Build history of the part. All positions in model axes, mm. Coordinates: 2 decimals unless noted, no trailing zeros. Loops run counter-clockwise (first coordinate to the right, second up) from the corner with the lowest first, then second, coordinate; pieces in that order, holes last.
Item 1: Flat gauge pins, fed straight in: pin 1 (1 mm diameter, centred on y = -147.5, z = -5.5, fed in from +X); pin 2 (1.8 mm diameter, centred on x = 0, y = -15, fed in from -Z); pin 3 (2 mm diameter, centred on y = -137, z = 10.5, fed in from -X); pin 4 (21 mm diameter, centred on x = 0, z = 0, fed in from +Y). Where does each tip first touch, or does it go through?
Item 2: Drill centre lines: line 1 along X through (y, z) = (-593.5, -1); line 2 along Y through (x, z) = (0, -18.6); line 3 along Z through (x, y) = (-2, -112) (3 decimals). Where is each one in solid material? Low to high.
Item 3: Cut at B-B (x = -11). List the corners of the cut face in (y, z).
Item 4: Cut at A-A (z = 11). List the corners of the cut face in (x, y).
Item 5: Mould opens along X. For faces 1 (the face through (-15.12, -325.38, -11.59)), 2 (the face through (17, 0, -6)), 3 (the face through (-3.783, -325.38, -17.035)) say: released by +X, released by -X, zero draft, split by the parting line, or undercut.
Item 6: Cut at C-C (y = -506.5). List the corners of the cut face in (x, z).
from build123d import *

# Parameters (mm, degrees)
F0_R     = 19.05
F0_R_2   = 17.45
F1_DEPTH = 660
F2_R     = 3.5625283299
F3_DEPTH = 20.050000094
F4_R     = 1
F5_DEPTH = 20.050000107


with BuildPart() as f1:
    # F0 (on Front) → F1 (new body)
    with BuildSketch(Plane.XZ):
        Circle(F0_R)
        Circle(F0_R_2, mode=Mode.SUBTRACT)
    extrude(amount=F1_DEPTH)

    # F2 (on Top) → F3 (cut, up to face)
    with BuildSketch(Plane.XY):
        with Locations((0, -140)):
            Circle(F2_R)
    extrude(amount=F3_DEPTH, mode=Mode.SUBTRACT)

    # F4 (on Top) → F5 (cut, up to face)
    with BuildSketch(Plane.XY):
        with Locations((0, -15)):
            Circle(F4_R)
    extrude(amount=-F5_DEPTH, mode=Mode.SUBTRACT)


solid = f1.part
Filled sheet:
1. pin 1: stops at x = 18.38
1. pin 2: stops at z = 17.43
1. pin 3: stops at x = -16.51
1. pin 4: passes through
2. line 1: x = -19.02 to -17.42, 17.42 to 19.02
2. line 2: y = -660 to -16, -14 to 0
2. line 3: z = -18.945 to -17.335, 17.335 to 18.945
3. outline: (-660, -15.55) - (0, -15.55) - (0, -13.55) - (-660, -13.55) - close; (-660, 13.55) - (0, 13.55) - (0, 15.55) - (-660, 15.55) - close
4. outline: (-15.55, -660) - (-13.55, -660) - (-13.55, 0) - (-15.55, 0) - close; (13.55, -660) - (15.55, -660) - (15.55, 0) - (13.55, 0) - close
5. face 1: split by the parting line
5. face 2: zero draft
5. face 3: undercut
6. outline: circle Ø38.1 at (0, 0); hole circle Ø34.9 at (0, 0)
